Geometry: final body of the model. Coordinates: model frame, mm. A direction names the side the tool comes from. Give positions to 0.01 mm unless a question says otherwise; leave off trailing zeros. Loops run counter-clockwise (first coordinate to the right, second up) from the corner with the lowest first, then second, coordinate; pieces in that order, holes last. Notation, with made-up numbers: (32.25, 75.25) - (72.25, 75.25) arc R9 ccw to (72.25, 85.25) - close; hole circle Ø6 at (53, -33). An arc over 180 degrees is marked (long way). Answer in a Markdown table with one row per item.
from build123d import *

# Parameters (mm, degrees)
SKETCH1_R           = 17.78
BOSS_EXTRUDE1_DEPTH = 100
SHELL1_T            = 2
CUT_EXTRUDE1_START  = 20
SKETCH2_W           = 4.427976762
SKETCH2_H           = 104.269834735
CUT_EXTRUDE1_DEPTH  = 5
SKETCH4_R           = 16.51
BOSS_EXTRUDE2_DEPTH = 20
SKETCH7_R           = 14.953216008
CUT_EXTRUDE4_DEPTH  = 32
SKETCH8_W           = 2.785852998
SKETCH8_H           = 3.149177074
SKETCH8_W_2         = 3.149177073
SKETCH8_H_2         = 3.205412378
SKETCH8_H_3         = 3.711530123
CUT_EXTRUDE5_DEPTH  = 104.112835283
BOSS_EXTRUDE4_DEPTH = 2


with BuildPart() as part:
    # Sketch1 → Boss-Extrude1 (new body)
    with BuildSketch(Plane(origin=(0, 0, 0), x_dir=(1, 0, 0), z_dir=(0, 1, 0))):
        with Locations(Location((0, 0, 0), (0, 0, 90))):
            Circle(SKETCH1_R)
    extrude(amount=BOSS_EXTRUDE1_DEPTH)

    # Shell1 (no face opened: a closed hollow body)
    add(offset(amount=-SHELL1_T, mode=Mode.PRIVATE), mode=Mode.SUBTRACT)

    # Sketch2 → Cut-Extrude1 (cut, symmetric)
    with BuildSketch(Plane(origin=(0, 0, 0), x_dir=(0, 0, -1), z_dir=(1, 0, 0)).offset(CUT_EXTRUDE1_START)):
        with Locations((0, 52.134917368)):
            Rectangle(SKETCH2_W, SKETCH2_H)
    extrude(amount=CUT_EXTRUDE1_DEPTH, both=True, mode=Mode.SUBTRACT)

    # Sketch4 → Boss-Extrude2 (add)
    with BuildSketch(Plane.XZ):
        with Locations(Location((0, 0, 0), (0, 0, 7.706571309))):
            Circle(SKETCH4_R)
    extrude(amount=BOSS_EXTRUDE2_DEPTH)

    # Sketch7 → Cut-Extrude4 (cut)
    with BuildSketch(Plane(origin=(0, -20, 0), x_dir=(-1, 0, 0), z_dir=(0, -1, 0))):
        with Locations(Location((0, 0, 0), (0, 0, 90))):
            Circle(SKETCH7_R)
    extrude(amount=-CUT_EXTRUDE4_DEPTH, mode=Mode.SUBTRACT)

    # Sketch8 → Cut-Extrude5 (cut, through all)
    with BuildSketch(Plane(origin=(0, 0, 0), x_dir=(1, 0, 0), z_dir=(0, 1, 0))):
        with Locations((0, 15.774003019)):
            Rectangle(SKETCH8_W, SKETCH8_H)
        with Locations((15.845399854, 0)):
            Rectangle(SKETCH8_W_2, SKETCH8_H_2)
        with Locations((0, -16.055179544)):
            Rectangle(SKETCH8_W, SKETCH8_H_3)
        with Locations((-15.845399854, 0)):
            Rectangle(SKETCH8_W_2, SKETCH8_H_2)
    extrude(amount=-CUT_EXTRUDE5_DEPTH, mode=Mode.SUBTRACT)

    # Sketch9 → Boss-Extrude4 (add)
    with BuildSketch(Plane.XZ.offset(20)):
        with BuildLine():
            ThreePointArc((16.14116018, 5.756014083), (12.168131115, 12.163725441), (5.760419757, 16.136754506))
            ThreePointArc((5.760419757, 16.136754506), (4.92620467, 15.722665224), (5.340293953, 14.888450137))
            ThreePointArc((5.340293953, 14.888450137), (11.236796189, 11.232390515), (14.892855811, 5.335888279))
            ThreePointArc((14.892855811, 5.335888279), (15.727070898, 4.921798996), (16.14116018, 5.756014083))
        make_face()
        with BuildLine():
            ThreePointArc((16.14116018, -5.756014083), (12.168131115, -12.163725441), (5.760419757, -16.136754506))
            ThreePointArc((5.760419757, -16.136754506), (4.92620467, -15.722665224), (5.340293953, -14.888450137))
            ThreePointArc((5.340293953, -14.888450137), (11.236796189, -11.232390515), (14.892855811, -5.335888279))
            ThreePointArc((14.892855811, -5.335888279), (15.727070898, -4.921798996), (16.14116018, -5.756014083))
        make_face()
        with BuildLine():
            ThreePointArc((-16.14116018, -5.756014083), (-12.168131115, -12.163725441), (-5.760419757, -16.136754506))
            ThreePointArc((-5.760419757, -16.136754506), (-4.92620467, -15.722665224), (-5.340293953, -14.888450137))
            ThreePointArc((-5.340293953, -14.888450137), (-11.236796189, -11.232390515), (-14.892855811, -5.335888279))
            ThreePointArc((-14.892855811, -5.335888279), (-15.727070898, -4.921798996), (-16.14116018, -5.756014083))
        make_face()
        with BuildLine():
            ThreePointArc((-16.14116018, 5.756014083), (-12.168131115, 12.163725441), (-5.760419757, 16.136754506))
            ThreePointArc((-5.760419757, 16.136754506), (-4.92620467, 15.722665224), (-5.340293953, 14.888450137))
            ThreePointArc((-5.340293953, 14.888450137), (-11.236796189, 11.232390515), (-14.892855811, 5.335888279))
            ThreePointArc((-14.892855811, 5.335888279), (-15.727070898, 4.921798996), (-16.14116018, 5.756014083))
        make_face()
    extrude(amount=-BOSS_EXTRUDE4_DEPTH)


solid = part.part
Q1. Cut plane C-C (x = 0). Output: boundary loops of the cut face in (y, z).
Check values:
| item | result |
|---|---|
| outline | (0, -17.78) - (100, -17.78) - (100, 17.78) - (0, 17.78) - (0, 14.95) - (2, 14.95) - (2, 15.78) - (98, 15.78) - (98, -15.78) - (2, -15.78) - (2, -14.95) - (0, -14.95) - close |
Q2. Reachability of faces 1 (the cylindrical face through (12.24, -19.01, 12.09)), 2 (the flat face through (12, -18, 12)), 3 (the cylindrical face through (4.492, -9.154, -14.263)) from +Z, -Z, +X, -X, +Y, -Y: full face, straight path, thin tool, end or side. Return the list, or none.
Check values:
| item | result |
|---|---|
| face 1 | +Z, +X, -Y |
| face 2 | +Z, +X |
| face 3 | -Y |
Q3. Cut plane D-D (z = 11). Output: boundary loops of the cut face in (x, y), and give its area (3 significant figures).
Check values:
| item | result |
|---|---|
| outline | (-13.97, 0) - (-12.31, 0) - (-12.31, -18) - (-13.23, -18) - (-13.23, -20) - (-10.13, -20) - (-10.13, 2) - (-11.31, 2) - (-11.31, 98) - (11.31, 98) - (11.31, 2) - (10.13, 2) - (10.13, -20) - (13.23, -20) - (13.23, -18) - (12.31, -18) - (12.31, 0) - (13.97, 0) - (13.97, 100) - (-13.97, 100) - close |
| area | 672 mm² |
Q4. First-contact query: pin 1 (1 mm diameter, centred on y = 0.5, z = 0.5, fed in from +X); pin 2 (12 mm diameter, centred on y = 79, z = -14, fed in from +X); pin 3 (1 mm diameter, centred on y = 84, z = -13, fed in from -X). Flat tips, straight axial feed; report the tip coordinate or a pass-through.
Check values:
| item | result |
|---|---|
| pin 1 | x = 15 |
| pin 2 | x = 15.88 |
| pin 3 | x = -12.64 |
Q5. Cut plane B-B (y = -11.5). Output: boundary loops of the cut face in (x, z), and give its area (3 significant figures).
Check values:
| item | result |
|---|---|
| outline | (-16.43, -1.6) arc R16.51 ccw to (-1.39, -16.45) - (-1.39, -14.89) arc R14.95 cw to (-14.87, -1.6) - close; (-16.43, 1.6) - (-14.87, 1.6) arc R14.95 cw to (-1.39, 14.89) - (-1.39, 16.45) arc R16.51 ccw to start; (1.39, -16.45) arc R16.51 ccw to (16.43, -1.6) - (14.87, -1.6) arc R14.95 cw to (1.39, -14.89) - close; (1.39, 14.89) arc R14.95 cw to (14.87, 1.6) - (16.43, 1.6) arc R16.51 ccw to (1.39, 16.45) - close |
| area | 135 mm² |
Q6. Draft query along Y for faces 4 (the flat face through (0, 100, 0)), 5 (the flat face through (11, -20, 11)), 6 (the cylindrical face through (-15.766, 49.328, -0.663)), 7 (the cylindrical face through (12.24, -19.01, -12.09)). Return one class per face: pulls with the +Y half, pulls with the -Y half, needs draft (parallel to the pull), parting line crosses it, or undercut.
Check values:
| item | result |
|---|---|
| face 4 | pulls with the +Y half |
| face 5 | pulls with the -Y half |
| face 6 | undercut |
| face 7 | needs draft |
Q7. Material intervals for line 1 along Z through (x, y) = (0, 48); line 2 along X through (y, z) = (31, 9); line 3 along X through (y, z) = (51, 0), sorted ascending.
Check values:
| item | result |
|---|---|
| line 1 | -17.78 to -15.78, 15.78 to 17.78 |
| line 2 | -15.33 to -12.96, 12.96 to 15.33 |
| line 3 | -17.78 to -15.78 |
Q8. Cut plane A-A (z = 0). Output: boundary loops of the cut face in (x, y), and give its area (3 significant figures).
Check values:
| item | result |
|---|---|
| outline | (-17.78, 0) - (-14.95, 0) - (-14.95, 2) - (-15.78, 2) - (-15.78, 98) - (15, 98) - (15, 100) - (-17.78, 100) - close; (14.95, 0) - (15, 0) - (15, 2) - (14.95, 2) - close |
| area | 263 mm² |
